Design review of the part built by this model. Coordinates are the model's own, in mm. Give positions to 0.01 mm unless a question says otherwise; leave off trailing zeros. Order: outer loops, then holes, each group sorted by start corner. A loop starts at its lowest first (then second) coordinate and runs counter-clockwise, first axis right, second up. Notation, with made-up numbers: M 60.25,40.25 L 74.25,40.25 A19 ccw 74.25,55.25 Z; hole C 53,18.25 d4. An arc over 180 degrees is marked long. Answer as a JSON object with one key per item and string values.
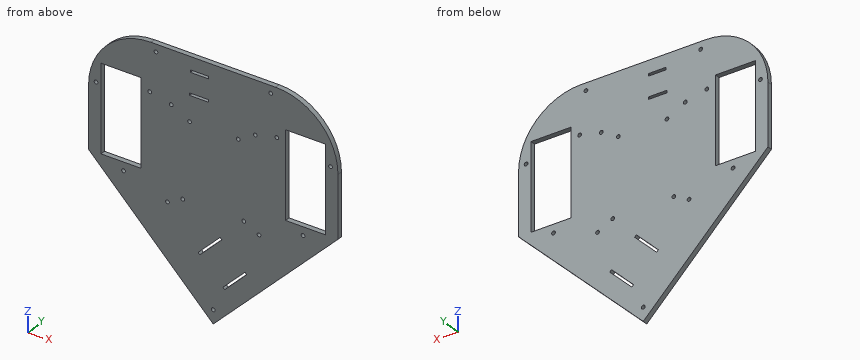
from build123d import *

# Parameters (mm, degrees)
BASIS_GRONDPLAAT_DEPTH = 4
WIELGATEN_SCHETS_W     = 32
WIELGATEN_SCHETS_H     = 70
WIELGATEN_DEPTH        = 10
BOORGAT1_SCHETS_R      = 1.5
BOORGAT1_DEPTH         = 181.321934329
SKETCH1_R              = 1.5
SKETCH1_W              = 15
SKETCH1_H              = 2
SKETCH1_W_2            = 14.4
CUT_EXTRUDE1_DEPTH     = 10
SKETCH2_R              = 1.5
CUT_EXTRUDE2_DEPTH     = 10


with BuildPart() as part:
    # basis_grondplaat_schets → basis_grondplaat (new body)
    with BuildSketch(Plane(origin=(0, 0, 0), x_dir=(1, 0, 0), z_dir=(0, 1, 0))):
        with BuildLine():
            Line((-50, -50), (50, -50))
            ThreePointArc((50, -50), (85.355339059, -35.355339059), (100, 0))
            Line((100, 0), (100, 50))
            Line((100, 50), (0, 150))
            Line((0, 150), (-100, 50))
            Line((-100, 50), (-100, 0))
            ThreePointArc((-100, 0), (-85.355339059, -35.355339059), (-50, -50))
        make_face()
    extrude(amount=BASIS_GRONDPLAAT_DEPTH)

    # wielgaten_schets → wielgaten (cut)
    with BuildSketch(Plane(origin=(0, 4, 0), x_dir=(1, 0, 0), z_dir=(0, 1, 0))):
        with Locations((-74, 15)):
            Rectangle(WIELGATEN_SCHETS_W, WIELGATEN_SCHETS_H)
    wielgaten = extrude(amount=-WIELGATEN_DEPTH, mode=Mode.SUBTRACT)

    # boorgat1_schets → boorgat1 (cut, through all)
    with BuildSketch(Plane.XZ):
        with Locations(Location((-46, 44, 0), (0, 0, 270))):
            Circle(BOORGAT1_SCHETS_R)
    extrude(amount=-BOORGAT1_DEPTH, mode=Mode.SUBTRACT)

    # Mirror1: wielgaten across plane
    add(wielgaten.mirror(Plane(origin=(0, 0, 0), x_dir=(0, 0, 1), z_dir=(1, 0, 0))), mode=Mode.SUBTRACT)

    # Sketch1 → Cut-Extrude1 (cut)
    with BuildSketch(Plane(origin=(0, 0, 0), x_dir=(-1, 0, 0), z_dir=(0, -1, 0))):
        with Locations(Location((-46, -44, 0), (0, 0, 90))):
            Circle(SKETCH1_R)
        with Locations(Location((-94, -4, 0), (0, 0, 90))):
            Circle(SKETCH1_R)
        with Locations(Location((94, -4, 0), (0, 0, 90))):
            Circle(SKETCH1_R)
        with Locations(Location((0, 139, 0), (0, 0, 90))):
            Circle(SKETCH1_R)
        with Locations(Location((24.5, 62.2, 0), (0, 0, 90))):
            Circle(SKETCH1_R)
        with Locations(Location((-24.5, 62.2, 0), (0, 0, 90))):
            Circle(SKETCH1_R)
        with Locations(Location((-20, 0.5, 0), (0, 0, 90))):
            Circle(SKETCH1_R)
        with Locations(Location((19, 0.5, 0), (0, 0, 90))):
            Circle(SKETCH1_R)
        Polygon((10.751885446, 100.378121725), (-6.925784083, 82.700452195), (-5.511570521, 81.286238633), (12.166099009, 98.963908163), align=None)
        Polygon((-25.45198175, 101.226649863), (-7.774312221, 118.904319392), (-9.188525783, 120.318532955), (-26.866195313, 102.640863425), align=None)
        with Locations((11.5, -20.75)):
            Rectangle(SKETCH1_W, SKETCH1_H)
        with Locations((11.2, -38.75)):
            Rectangle(SKETCH1_W_2, SKETCH1_H)
    extrude(amount=-CUT_EXTRUDE1_DEPTH, mode=Mode.SUBTRACT)

    # Sketch2 → Cut-Extrude2 (cut)
    with BuildSketch(Plane(origin=(0, 0, 0), x_dir=(-1, 0, 0), z_dir=(0, -1, 0))):
        with Locations(Location((51, -11.5, 0), (0, 0, 90))):
            Circle(SKETCH2_R)
        with Locations(Location((33.7, -7.5, 0), (0, 0, 90))):
            Circle(SKETCH2_R)
        with Locations(Location((-33.7, -7.5, 0), (0, 0, 90))):
            Circle(SKETCH2_R)
        with Locations(Location((-51, -11.5, 0), (0, 0, 90))):
            Circle(SKETCH2_R)
        with Locations(Location((36.7, 68.5, 0), (0, 0, 90))):
            Circle(SKETCH2_R)
        with Locations(Location((-36.7, 68.5, 0), (0, 0, 90))):
            Circle(SKETCH2_R)
        with Locations(Location((-72, 56.75, 0), (0, 0, 90))):
            Circle(SKETCH2_R)
        with Locations(Location((72, 56.75, 0), (0, 0, 90))):
            Circle(SKETCH2_R)
    extrude(amount=-CUT_EXTRUDE2_DEPTH, mode=Mode.SUBTRACT)


solid = part.part
(1) We need section A-A (x = -80). Write out the cut boundary in (y, z), plus the area to 3 significant figures.
Checked values:
{"outline": "M 0,-70 L 4,-70 L 4,-50 L 0,-50 Z; M 0,20 L 4,20 L 4,40 L 0,40 Z", "area": "160 mm^2"}
(2) Insertion check: pin 1 (0.6 mm diameter, centred on y = 3, z = 39, fed in from -X); pin 2 (1.8 mm diameter, centred on x = -46, z = 44, fed in from -Y); pin 3 (2 mm diameter, centred on y = 2.5, z = -87.5, fed in from +X); pin 4 (1.5 mm diameter, centred on y = 3, z = -77, fed in from -X). Each pin has a flat end and moves straight along its axis. Give the tip position at first contact, or say it passes through.
Checked values:
{"pin 1": "stops at x = -81.66", "pin 2": "passes through", "pin 3": "stops at x = 63.5", "pin 4": "stops at x = -73.75"}
(3) We need section B-B (z = -47). Write out the cut boundary in (x, y), plus the area to 3 significant figures.
Checked values:
{"outline": "M -100,0 L -90,0 L -90,4 L -100,4 Z; M -58,0 L 58,0 L 58,4 L -58,4 Z; M 90,0 L 100,0 L 100,4 L 90,4 Z", "area": "544 mm^2"}
(4) To check wall thickness, follow L1, parallel to X at y = 2.9, z = -0.5; L2, parallel to X at y = 2.8, z = -9; L3, parallel to X at y = 3.45, z = 8.5. State the ranges of each line that lie inside material, in increasing order. Write a range as from..to.
Checked values:
{"L1": "x = -100..-90, -58..-20.5, -17.5..18.5, 21.5..58, 90..100", "L2": "x = -100..-90, -58..58, 90..100", "L3": "x = -99.27..-90, -58..-34.82, -32.58..32.58, 34.82..58, 90..99.27"}
(5) We need section C-C (y = 2.3). Count the separate pieces of the cut face and the enclosed holes in it, plus the area to 3 significant figures.
Checked values:
{"separate pieces": "1", "enclosed holes": "23", "area": "24,200 mm^2"}
(6) We need section D-D (z = 16). Write out the cut boundary in (x, y), plus the area to 3 significant figures.
Checked values:
{"outline": "M -97.37,0 L -90,0 L -90,4 L -97.37,4 Z; M -58,0 L 58,0 L 58,4 L -58,4 Z; M 90,0 L 97.37,0 L 97.37,4 L 90,4 Z", "area": "523 mm^2"}
